from build123d import *

# Parameters (mm, degrees)
BOSS_EXTRUDE1_DEPTH   = 100
CHAMFER1_SIZE         = 0.5
CHAMFER1_SIZE2        = 0.288675135
CHAMFER1_PART_2_SIZE  = 0.5
CHAMFER1_PART_2_SIZE2 = 0.288675135
CHAMFER1_PART_3_SIZE  = 0.5
CHAMFER1_PART_3_SIZE2 = 0.288675135
CHAMFER1_PART_4_SIZE  = 0.5
CHAMFER1_PART_4_SIZE2 = 0.288675135
SKETCH2_R             = 1.75
CUT_EXTRUDE1_DEPTH    = 8
SKETCH3_R             = 3
CUT_EXTRUDE2_DEPTH    = 4.5
LPATTERN1_COUNT       = 8
LPATTERN1_PITCH       = 25


with BuildPart() as part:
    # Sketch1 → Boss-Extrude1 (new body, symmetric)
    with BuildSketch(Plane.XY):
        with BuildLine():
            Line((-6, -4), (6, -4))
            Line((6, -4), (6, 0.3))
            ThreePointArc((6, 0.3), (4.8, 1.5), (6, 2.7))
            Line((6, 2.7), (6, 4))
            Line((6, 4), (-6, 4))
            Line((-6, 4), (-6, 2.7))
            ThreePointArc((-6, 2.7), (-4.8, 1.5), (-6, 0.3))
            Line((-6, 0.3), (-6, -4))
        make_face()
    extrude(amount=BOSS_EXTRUDE1_DEPTH, both=True)

    # Chamfer1
    chamfer1_edges = [part.edges().sort_by_distance(p)[0] for p in [
        (6, -4, 0),
    ]]
    chamfer1_side = [part.faces().sort_by_distance(p)[0] for p in [
        (0, -4, 0),
    ]]
    chamfer(chamfer1_edges, length=CHAMFER1_SIZE, length2=CHAMFER1_SIZE2, reference=chamfer1_side[0])

    # Chamfer1 part 2
    chamfer1_part_2_edges = [part.edges().sort_by_distance(p)[0] for p in [
        (-6, -4, 0),
    ]]
    chamfer1_part_2_side = [part.faces().sort_by_distance(p)[0] for p in [
        (-6, -1.85, 0),
    ]]
    chamfer(chamfer1_part_2_edges, length=CHAMFER1_PART_2_SIZE, length2=CHAMFER1_PART_2_SIZE2, reference=chamfer1_part_2_side[0])

    # Chamfer1 part 3
    chamfer1_part_3_edges = [part.edges().sort_by_distance(p)[0] for p in [
        (-6, 4, 0),
    ]]
    chamfer1_part_3_side = [part.faces().sort_by_distance(p)[0] for p in [
        (0, 4, 0),
    ]]
    chamfer(chamfer1_part_3_edges, length=CHAMFER1_PART_3_SIZE, length2=CHAMFER1_PART_3_SIZE2, reference=chamfer1_part_3_side[0])

    # Chamfer1 part 4
    chamfer1_part_4_edges = [part.edges().sort_by_distance(p)[0] for p in [
        (6, 4, 0),
    ]]
    chamfer1_part_4_side = [part.faces().sort_by_distance(p)[0] for p in [
        (6, 3.35, 0),
    ]]
    chamfer(chamfer1_part_4_edges, length=CHAMFER1_PART_4_SIZE, length2=CHAMFER1_PART_4_SIZE2, reference=chamfer1_part_4_side[0])

    # Sketch2 → Cut-Extrude1 (cut)
    with BuildSketch(Plane(origin=(0, 4, 0), x_dir=(1, 0, 0), z_dir=(0, 1, 0))):
        with Locations((0.092454629, -87.5)):
            Circle(SKETCH2_R)
    cut_extrude1 = extrude(amount=-CUT_EXTRUDE1_DEPTH, mode=Mode.SUBTRACT)

    # Sketch3 → Cut-Extrude2 (cut)
    with BuildSketch(Plane(origin=(0, 4, 0), x_dir=(1, 0, 0), z_dir=(0, 1, 0))):
        with Locations((0.092454629, -87.5)):
            Circle(SKETCH3_R)
    cut_extrude2 = extrude(amount=-CUT_EXTRUDE2_DEPTH, mode=Mode.SUBTRACT)

    # LPattern1: Cut-Extrude1, Cut-Extrude2 ×8
    with Locations(*[(0, 0, -i * LPATTERN1_PITCH) for i in range(1, LPATTERN1_COUNT)]):
        add(cut_extrude1, mode=Mode.SUBTRACT)
        add(cut_extrude2, mode=Mode.SUBTRACT)


solid = part.part
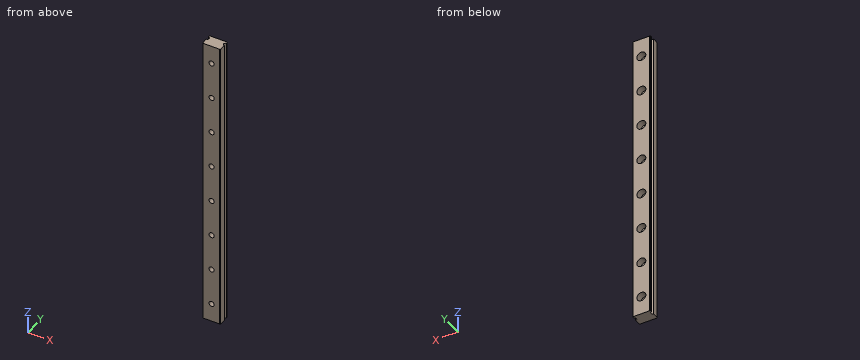
Could you check a few things on this model? Use its own coordinates, in mm. Give positions to 0.01 mm unless a question says otherwise; leave off trailing zeros. Order: outer loops, then holes, each group sorted by start corner. A loop starts at its lowest first (then second) coordinate and runs counter-clockwise, first axis right, second up.
Item 1: If we section it at A-A, the plane y = 1.5: Count the separate pieces of the cut face and the enclosed holes in it, plus the area to 3 significant figures.
Item 2: If we section it at B-B, the plane z = 37.5: Write out the boundary of the cut face in (x, y).
Item 3: I'm going to push flat-ended pins straight in: pin 1 (1 mm diameter, centred on y = 2, z = 4.5, fed in from +X); pin 2 (3 mm diameter, centred on x = 1.5, z = 37.5, fed in from +Y); pin 3 (1 mm diameter, centred on x = -0.5, z = -63, fed in from +Y). Where does each tip first touch, or does it pass through?
Item 4: I need wall thicknesses on line 1 (X direction, y = -1.2, z = -37.5); line 2 (X direction, y = 1.5, z = 0); line 3 (X direction, y = 1.65, z = 12.5). Which ranges of each line are inside material? Lowest first, please.
Item 5: If we section it at C-C, the plane z = 76.5: Write out the boundary of the cut face in (x, y), plus the area to 3 significant figures.
Values:
1. separate pieces: 1
1. enclosed holes: 8
1. area: 1,690 mm2
2. outline: (-6, -3.5) - (-5.71, -4) - (-1.66, -4) - (-1.66, -0.5) - (-2.91, -0.5) - (-2.91, 4) - (-5.5, 4) - (-6, 3.71) - (-6, 2.7) arc R1.2 cw to (-6, 0.3) - close; (1.84, -4) - (5.5, -4) - (6, -3.71) - (6, 0.3) arc R1.2 cw to (6, 2.7) - (6, 3.5) - (5.71, 4) - (3.09, 4) - (3.09, -0.5) - (1.84, -0.5) - close
3. pin 1: stops at x = 5.34
3. pin 2: stops at y = -0.5
3. pin 3: passes through
4. line 1: x = -6 to -1.66, 1.84 to 6
4. line 2: x = -4.8 to 4.8
4. line 3: x = -4.81 to -2.91, 3.09 to 4.81
5. outline: (-6, -3.5) - (-5.71, -4) - (5.5, -4) - (6, -3.71) - (6, 0.3) arc R1.2 cw to (6, 2.7) - (6, 3.5) - (5.71, 4) - (-5.5, 4) - (-6, 3.71) - (-6, 2.7) arc R1.2 cw to (-6, 0.3) - close
5. area: 91.2 mm2
